```python
from build123d import *

# Parameters (mm, degrees)
EXTRUDE_1_DEPTH   = 10
EXTRUDE_1_2_DEPTH = 10
SKETCH_2_3_R      = 26
SKETCH_2_3_R_2    = 8
SKETCH_2_3_R_3    = 4
SKETCH_2_3_R_4    = 65
EXTRUDE_2_DEPTH   = 20


with BuildPart() as part:
    # Sketch 2 → Extrude 1 (new body)
    with BuildSketch(Plane.XY):
        with BuildLine():
            ThreePointArc((-59.707166842, 60.765834645), (-48.770005737, 53.957911858), (-50.302314794, 41.166456325))
            ThreePointArc((-50.302314794, 41.166456325), (-11.477303942, 63.978679997), (32.856212496, 56.084483598))
            ThreePointArc((32.856212496, 56.084483598), (-73.921140449, 80.079620615), (-174.861132012, 37.791468547))
            ThreePointArc((-174.861132012, 37.791468547), (-152.986381903, 43.512029194), (-134.903213902, 29.93894769))
            ThreePointArc((-134.903213902, 29.93894769), (-135.536993635, 37.600652682), (-130.545808802, 43.448000294))
            ThreePointArc((-130.545808802, 43.448000294), (-96.126281422, 56.196575534), (-59.707166842, 60.765834645))
        make_face()
    extrude(amount=EXTRUDE_1_DEPTH)



with BuildPart() as body_2:
    # Sketch 2 → Extrude 1 2 (new body)
    with BuildSketch(Plane.XY):
        with BuildLine():
            Line((-66.371369906, -65), (0, -65))
            ThreePointArc((0, -65), (-30.089153243, -57.616341928), (-53.342367432, -37.142857143))
            ThreePointArc((-53.342367432, -37.142857143), (-53.013600163, -42.314550249), (-57.445626465, -45))
            Line((-57.445626465, -45), (-61.719917869, -45))
            ThreePointArc((-61.719917869, -45), (-65.741068408, -43.915948839), (-68.67243572, -40.957587084))
            Line((-68.67243572, -40.957587084), (-98.206043194, 10.925777398))
            ThreePointArc((-98.206043194, 10.925777398), (-103.335935989, 16.102910468), (-110.372949433, 18))
            Line((-110.372949433, 18), (-127.405882918, 18))
            ThreePointArc((-127.405882918, 18), (-130.643763547, 19.18999619), (-132.340417932, 22.193548387))
            ThreePointArc((-132.340417932, 22.193548387), (-132.085244225, 20.103671341), (-132, 18))
            ThreePointArc((-132, 18), (-134.644933514, 6.574551675), (-142.04160534, -2.526315789))
            ThreePointArc((-142.04160534, -2.526315789), (-138.569506528, -0.649136365), (-134.676192421, 0))
            Line((-134.676192421, 0), (-121.977178056, 0))
            ThreePointArc((-121.977178056, 0), (-115.945452247, -1.626076742), (-111.54840128, -6.063619373))
            Line((-111.54840128, -6.063619373), (-83.752664534, -54.893967711))
            ThreePointArc((-83.752664534, -54.893967711), (-76.424246255, -62.289872096), (-66.371369906, -65))
        make_face()
    extrude(amount=EXTRUDE_1_2_DEPTH)


with BuildPart() as part_1:
    add(part.part)

    add(body_2.part)  # Extrude 2 merges body 2
    # Sketch 2_3 → Extrude 2 (add)
    # profile 1 of 2: a face of its own
    with BuildSketch(Plane.XY):
        with Locations(Location((-158, 18, 0), (0, 0, 130.428983745))):
            Circle(SKETCH_2_3_R)
        with Locations((-158, 18)):
            Circle(SKETCH_2_3_R_2, mode=Mode.SUBTRACT)
        with Locations((-170.02081528, 5.97918472)):
            Circle(SKETCH_2_3_R_3, mode=Mode.SUBTRACT)
        with Locations((-145.97918472, 5.97918472)):
            Circle(SKETCH_2_3_R_3, mode=Mode.SUBTRACT)
        with Locations((-145.97918472, 30.02081528)):
            Circle(SKETCH_2_3_R_3, mode=Mode.SUBTRACT)
        with Locations((-170.02081528, 30.02081528)):
            Circle(SKETCH_2_3_R_3, mode=Mode.SUBTRACT)
    # profile 2 of 2: a face of its own
    with BuildSketch(Plane.XY):
        with Locations(Location((0, 0, 0), (0, 0, 214.849904579))):
            Circle(SKETCH_2_3_R_4)
        with BuildLine():
            ThreePointArc((-21.846902457, 7.19116493), (-23, 0), (-21.846902457, -7.19116493))
            Line((-21.846902457, -7.19116493), (-37.238903997, -14.603562205))
            ThreePointArc((-37.238903997, -14.603562205), (-36.038754716, -17.355349565), (-34.635601563, -20.009375412))
            Line((-34.635601563, -20.009375412), (-19.243600022, -12.596978138))
            ThreePointArc((-19.243600022, -12.596978138), (-14.340265443, -17.982124097), (-7.999041746, -21.564214132))
            Line((-7.999041746, -21.564214132), (-11.800552187, -38.219719623))
            ThreePointArc((-11.800552187, -38.219719623), (-8.900837358, -38.997116487), (-5.950984714, -39.554845227))
            Line((-5.950984714, -39.554845227), (-2.149474273, -22.899339736))
            ThreePointArc((-2.149474273, -22.899339736), (5.117981481, -22.42334198), (11.87226055, -19.698970263))
            Line((11.87226055, -19.698970263), (22.523856108, -33.055648625))
            ThreePointArc((22.523856108, -33.055648625), (24.939592074, -31.273259299), (27.214845003, -29.314709814))
            Line((27.214845003, -29.314709814), (16.563249445, -15.958031452))
            ThreePointArc((16.563249445, -15.958031452), (20.722283962, -9.979326), (22.803508502, -3))
            Line((22.803508502, -3), (39.88734135, -3))
            ThreePointArc((39.88734135, -3), (40, 0), (39.88734135, 3))
            Line((39.88734135, 3), (22.803508502, 3))
            ThreePointArc((22.803508502, 3), (20.722283962, 9.979326), (16.563249445, 15.958031452))
            Line((16.563249445, 15.958031452), (27.214845003, 29.314709814))
            ThreePointArc((27.214845003, 29.314709814), (24.939592074, 31.273259299), (22.523856108, 33.055648625))
            Line((22.523856108, 33.055648625), (11.87226055, 19.698970263))
            ThreePointArc((11.87226055, 19.698970263), (5.117981481, 22.42334198), (-2.149474273, 22.899339736))
            Line((-2.149474273, 22.899339736), (-5.950984714, 39.554845227))
            ThreePointArc((-5.950984714, 39.554845227), (-8.900837358, 38.997116487), (-11.800552187, 38.219719623))
            Line((-11.800552187, 38.219719623), (-7.999041746, 21.564214132))
            ThreePointArc((-7.999041746, 21.564214132), (-14.340265443, 17.982124097), (-19.243600022, 12.596978138))
            Line((-19.243600022, 12.596978138), (-34.635601563, 20.009375412))
            ThreePointArc((-34.635601563, 20.009375412), (-36.038754716, 17.355349565), (-37.238903997, 14.603562205))
            Line((-37.238903997, 14.603562205), (-21.846902457, 7.19116493))
        make_face(mode=Mode.SUBTRACT)
    extrude(amount=EXTRUDE_2_DEPTH)


solid = part_1.part
```
Part model, mm, in its own coordinate system. A direction names the side the tool comes from. Round coordinates to 2 decimals unless told otherwise and drop trailing zeros. Write each loop counter-clockwise with the first axis right and the second up, starting at its lowest first coordinate (ties: lowest second). Pieces come first, ordered by that corner, then holes. Notation, with made-up numbers: (-21, 72) -> (21, 72) arc R28 cw to (21, 90) -> close; hole circle Ø10 at (23, 47.25). An arc over 180 degrees is marked (long way). Return JSON: item names as keys, results as strings. Group by question number.
Q1. Saw through at A-A on x = -158. Write the cut outline in (y, z).
Q2. Which spindle directions (+Z, -Z, +X, -X, +Y, -Y) get a long thin tool onto all of the face, cutting with end or side? Do faces 3 (the cylindrical face through (43.771, -48.053, 9.86)), 4 (the flat face through (-9.873, -29.775, 9.86)), 5 (the flat face through (-128, 0, 5)). Say none if no direction does.
Q3. Pin check, flat tips, straight feed: pin 1 (8 mm diameter, centred on x = -117, z = 4, fed in from +Y); pin 2 (5 mm diameter, centred on x = -170.02, y = 5.98, fed in from +Z); pin 3 (5 mm diameter, centred on y = 15, z = 11, fed in from +X); pin 4 (8 mm diameter, centred on x = -130, z = 3, fed in from -Y). Stop position of each tip, or through.
Q4. Mould opens along X. For faces 1 (the cylindrical face through (-138.622, -0.667, 4.93)), 2 (the flat face through (-15, 23, 20)) say: pulls with the +X half, pulls with the -X half, needs draft (parallel to the pull), parting line crosses it, or undercut.
Q5. Probe L1, parallel to X at y = 36.5, z = 10.75; L2, parallel to X at y = 7.5, z = 6.75; L3, parallel to Y at x = -170.5, z = 18.25. List the from-to ranges inside material, lowest first. Write a range as [from, to].
Q6. Saw through at C-C on z = 3. State how many separate pieces and enclosed holes the cut face has, plus the area to 3 significant figures.
Q7. Saw through at B-B on y = 52. Write the cut outline in (x, z), plus the area to 3 significant figures.
Answer:
{
 "1": {"outline": "(-8, 0) -> (10, 0) -> (10, 20) -> (-8, 20) -> close; (26, 0) -> (50.53, 0) -> (50.53, 10) -> (44, 10) -> (44, 20) -> (26, 20) -> close"},
 "2": {"face 3": "+Z", "face 4": "+Z, -Z", "face 5": "+Z, -Z, -Y"},
 "3": {"pin 1": "y = 72.21", "pin 2": "through", "pin 3": "x = 63.79", "pin 4": "y = 0"},
 "4": {"face 1": "undercut", "face 2": "needs draft"},
 "5": {"L1": "[-176.27, -139.73], [-53.78, -11.41], [-5.25, 53.78]", "L2": "[-181.79, -173.72], [-166.32, -149.68], [-142.28, -96.26], [-64.57, -22.49], [21.74, 64.57]", "L3": "[-4.8, 2.01], [9.95, 26.05], [33.99, 40.8]"},
 "6": {"separate pieces": "1", "enclosed holes": "7", "area": "18,600 mm2"},
 "7": {"outline": "(-155.75, 0) -> (-110.39, 0) -> (-110.39, 10) -> (-155.75, 10) -> close; (-48.03, 0) -> (39, 0) -> (39, 20) -> (-39, 20) -> (-39, 10) -> (-48.03, 10) -> close", "area": "2,100 mm2"}
}
